The model under review builds one solid part; all positions refer to its coordinate system, in mm. Round coordinates to 2 decimals unless told otherwise and drop trailing zeros. Write each loop counter-clockwise with the first axis right and the second up, starting at its lowest first coordinate (ties: lowest second). Pieces come first, ordered by that corner, then holes.
Item 1: To check wall thickness, follow L1, parallel to Y at x = 4, z = 0.2; L2, parallel to Y at x = 7.25, z = -0.9; L3, parallel to Y at x = 3, z = -1.3. State the ranges of each line that lie inside material, in increasing order.
Item 2: Add section A-A (z = 0). Give the boundary of the cut face in (x, y).
Item 3: Add section C-C (x = 3). Give the boundary of the cut face in (y, z), plus the area to 3 significant figures.
Item 4: Clearance check with a flat-ended pin moving along its axis: pin 1 Ø1.5 at (x, z) = (3, -1) entering from +Y. State where the tip first meets the part, or that it passes through.
Item 5: Add section B-B (y = 0). Give the boundary of the cut face in (x, z).
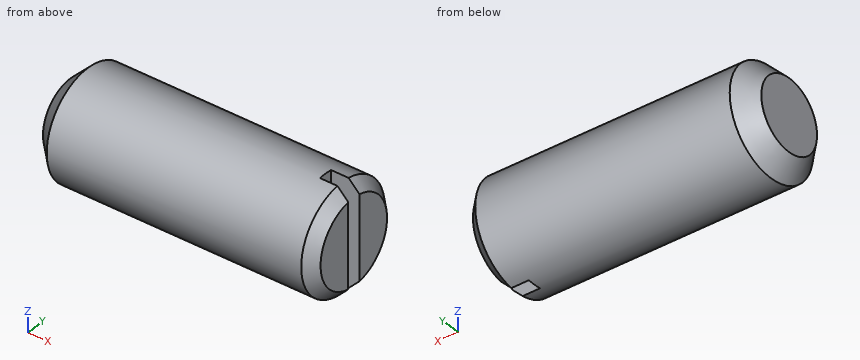
Autodesk Inventor part; units mm, degrees
ref_plane "Work Plane1" through (4, 0, 0) normal (0, 0, 1) x (1, 0, 0)
ref_plane "YZ Plane" through (0, 0, 0) normal (1, 0, 0) x (0, 1, 0)
ref_plane "XZ Plane" through (0, 0, 0) normal (0, 1, 0) x (-1, 0, 0)
sketch "Sketch1" plane through (0, 0, 0) normal (0, 0, 1) x (1, 0, 0)
  line L0 (0, 0) -> (8, 0)
  line L1 (8, 0) -> (8, 1.5)
  line L2 (8, 1.5) -> (0, 1.5)
  line L3 (0, -0.3) -> (0, 1.8)
  line L4 (0, 1.5) -> (0, 0)
  dimension "d0" = 3
  dimension "d2" = 8
revolve "Body" add sketch "Sketch1" angle 360 about axis through (0, 0, 0) along (1, 0, 0)
chamfer "Chamfer1" distance 0.3067 angle 45 1 edges at (8, -1.5, 0) measured on face at (8, -0.2885, 0.9187)
sketch "Sketch2" plane through (0, 0, 0) normal (0, 0, 1) x (1, 0, 0)
  line L0 (8, 1.1933) -> (8, -1.1933)
  line L1 (7.04, 0) -> (8.16, 0)
  line L2 (8, 0.2) -> (7.2, 0.2)
  line L3 (7.2, 0.2) -> (7.2, 0)
  line L4 (7.2, -0.2) -> (7.2, 0)
  line L5 (7.2, -0.2) -> (8, -0.2)
  dimension "d8" = 0.2
  dimension "d9" = 0.8
extrude "Slot1" cut sketch "Sketch2" against normal mid plane 3
thread "Thread"
chamfer "Chamfer2" distance 0.5 angle 45 1 edges at (0, -1.5, 0) measured on face at (2.5644, -0.6479, 1.3529)
ref_plane "Work Plane1" through (4, 0, 0) normal (0, 0, 1) x (1, 0, 0)
equation "\"d8\" = 0.5 * SBR"
equation "\"d9\" = STI"
equation "\"d10\" = NND"
equation "\"d3\" = -0.5 * GD1 + 0.5 * NND"
equation "\"d4\" = FAWI"
equation "\"d34\" = -0.5 * GD1 + 0.5 * NND"
equation "\"d5\" = NLG"
equation "\"d14\" = FAWI"
equation "\"d0\" = NND"
equation "\"d2\" = NLG"
equation "\"NND\" = 3"
equation "\"NLG\" = 8"
equation "\"FAWI\" = 45deg"
equation "\"GD1\" = THREADDIA - 1.2269 * PTC"
equation "\"FAWI1\" = 45deg"
equation "\"SPD\" = 2"
equation "\"SBR\" = 0.4"
equation "\"STI\" = 0.8"
equation "\"GUL\" = 0.61345 * PTC"
equation "\"THREADDIA\" = 3"
equation "\"TOA\" = 30deg"
equation "\"PTC\" = 0.5"
equation "\"GAL\" = 0.61345 * PTC"
properties part number "ISO 4766 - M3 x 8" material "Stainless Steel, 440C"
Numbers:
1. L1: y = -1.49 to 1.49
1. L2: y = -1.2 to -0.2, 0.2 to 1.2
1. L3: y = -0.75 to 0.75
2. outline: (0, -1) - (0.5, -1.5) - (7.69, -1.5) - (8, -1.19) - (8, -0.2) - (7.2, -0.2) - (7.2, 0.2) - (8, 0.2) - (8, 1.19) - (7.69, 1.5) - (0.5, 1.5) - (0, 1) - close
3. outline: circle Ø3 at (0, 0)
3. area: 7.07 mm2
4. pin 1: stops at y = 1.48
5. outline: (0, -1) - (0.5, -1.5) - (7.2, -1.5) - (7.2, 1.5) - (0.5, 1.5) - (0, 1) - close
